```python
from build123d import *

# Parameters (mm, degrees)
SALIENTE_EXTRUIR1_DEPTH  = 5
CORTE_CUCHILLA_START     = 29.061909686
CORTE_CUCHILLA_OUTLINE_W = 100
CORTE_CUCHILLA_OUTLINE_H = 11
CORTE_CUCHILLA_DEPTH     = 4.938090314


with BuildPart() as part:
    # Croquis2 → Saliente-Extruir1 (new body)
    with BuildSketch(Plane(origin=(0, 0, 0), x_dir=(1, 0, 0), z_dir=(0, 1, 0))):
        Polygon((-50, 1), (-50, 16), (-26, 16), (-26, 50), (26, 50), (26, 16), (50, 16), (50, 1), (26, 1), (26, -33), (50, -33), (50, -50), (-50, -50), (-50, -33), (-26, -33), (-26, 1), align=None)
    extrude(amount=SALIENTE_EXTRUIR1_DEPTH)

    # Corte-Cuchilla: read off the stored shape, not the designer's step
    # Corte-Cuchilla outline → Corte-Cuchilla (cut)
    with BuildSketch(Plane(origin=(0, 0, 0), x_dir=(1, 0, 0), z_dir=(0, 0.8137334712067352, 0.5812381937190961)).offset(CORTE_CUCHILLA_START)):
        with Locations((0, -36.5)):
            Rectangle(CORTE_CUCHILLA_OUTLINE_W, CORTE_CUCHILLA_OUTLINE_H)
    extrude(amount=CORTE_CUCHILLA_DEPTH, mode=Mode.SUBTRACT)


solid = part.part
```
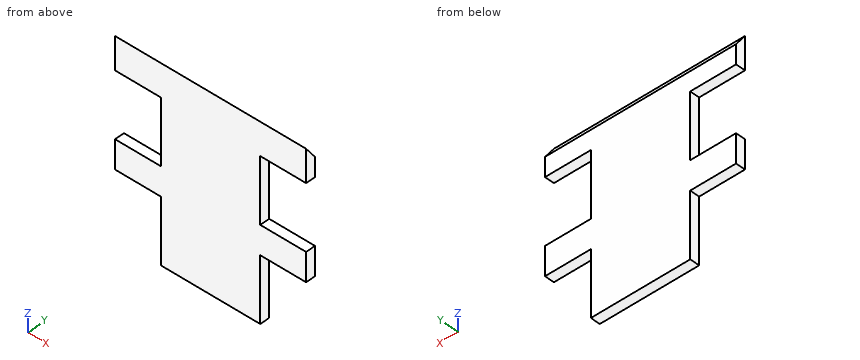
CAD build for the part. Positions are in the model's coordinates, mm. Round coordinates to 2 decimals unless told otherwise and drop trailing zeros. Order: outer loops, then holes, each group sorted by start corner. A loop starts at its lowest first (then second) coordinate and runs counter-clockwise, first axis right, second up. Notation, with made-up numbers: (60, 75.5) - (107, 75.5) arc R14 ccw to (107, 101.5) - close; hole circle Ø10 at (-12, 62.25). An arc over 180 degrees is marked (long way). Answer in a Markdown table with one row per item. Add a question column.
(1) Band-saw the part on B-B on y = 3.65. List the corners of the cut face in (x, z).
(2) Band-saw the part on C-C on z = -27. List the corners of the cut face in (x, y).
(3) Band-saw the part on D-D on z = 44.5. List the corners of the cut face in (x, y), and give its area (3 significant figures).
(4) Drop flat-ended pins along their axis: pin 1 Ø1 at (y, z) = (3.5, 32) entering from +X; pin 2 Ø1.5 at (x, y) = (33, 3) entering from +Z; pin 3 Ø2.5 at (y, z) = (3, -28.5) entering from -X. Give the stop position or say it passes through.
(5) Probe L1, parallel to X at y = 4.05, z = 30; L2, parallel to Z at x = -42, y = 0.35; L3, parallel to Z at x = -46, y = 0.55. List the from-to ranges inside material, lowest first. Write a range as [from, to].
(6) Band-saw the part on A-A on x = 30. List the corners of the cut face in (y, z).
Data:
| question | item | result |
|---|---|---|
| 1 | outline | (-50, -16) - (-26, -16) - (-26, -50) - (26, -50) - (26, -16) - (50, -16) - (50, -1) - (26, -1) - (26, 33) - (50, 33) - (50, 44.89) - (-50, 44.89) - (-50, 33) - (-26, 33) - (-26, -1) - (-50, -1) - close |
| 2 | outline | (-26, 0) - (26, 0) - (26, 5) - (-26, 5) - close |
| 3 | outline | (-50, 0) - (50, 0) - (50, 3.93) - (-50, 3.93) - close |
| 3 | area | 393 mm^2 |
| 4 | pin 1 | stops at x = 26 |
| 4 | pin 2 | stops at z = 46.85 |
| 4 | pin 3 | stops at x = -26 |
| 5 | L1 | x = [-26, 26] |
| 5 | L2 | z = [-16, -1], [33, 49.51] |
| 5 | L3 | z = [-16, -1], [33, 49.23] |
| 6 | outline | (0, -16) - (5, -16) - (5, -1) - (0, -1) - close; (0, 33) - (5, 33) - (5, 43) - (0, 50) - close |
